Part model, mm, in its own coordinate system. A direction names the side the tool comes from. Coordinates: 2 decimals unless noted, no trailing zeros. Loops run counter-clockwise (first coordinate to the right, second up) from the corner with the lowest first, then second, coordinate; pieces in that order, holes last. Notation, with made-up numbers: M 28.5,43 L 32.5,43 A20 cw 32.5,68 Z; hole C 87.5,-18 d9. An arc over 180 degrees is marked long. Use a Markdown table: item, result. Add a question column.
1) Pin check, flat tips, straight feed: pin 1 Ø24 at (y, z) = (-2.5, -3.5) entering from +X; pin 2 Ø0.6 at (x, z) = (0.5, 8.5) entering from +Y; pin 3 Ø8 at (x, z) = (37.5, 14.5) entering from +Y; pin 4 Ø1.5 at (y, z) = (2.5, 9.5) entering from +X. Stop position of each tip, or through.
2) Tool access for faces 4 (the flat face through (65, 62, 0)), 5 (the flat face through (1, 0, -11.75)), 6 (the cylindrical face through (51.25, 63.48, 14.96)): list every direction of +Z, -Z, +X, -X, +Y, -Y with a clear straight run to the whole face (end or side of a thin tool).
3) Wall check: probe 1 along Y at (x, z) = (72, 18.5); probe 2 along X at (y, z) = (-5, -14); probe 3 along X at (y, z) = (30.5, 7). Give the ranges that are in metal, low to high. Write a range as from..to.
4) Pull direction X, two halves, no side cores. Call faces 1 (the flat face through (20, 5, -18)), 2 (the cylindrical face through (1.48, -11.75, -10.04)), 3 (the cylindrical face through (51.25, 63.48, -15.04)): released by +X, released by -X, zero draft, split by the parting line, or undercut.
5) Band-saw the part on B-B (z = -10). List the corners of the cut face in (x, y), plus the area to 3 significant figures.
6) Band-saw the part on C-C (x = 69.5). List the corners of the cut face in (y, z).
7) Band-saw the part on D-D (z = -2). List the corners of the cut face in (x, y), plus the area to 3 significant figures.
8) Band-saw the part on A-A (y = 9). List the corners of the cut face in (x, z), plus the area to 3 significant figures.
from build123d import *

# Parameters (mm, degrees)
SKETCH_1_W            = 30
SKETCH_1_H            = 30
EXTRUDE_1_DEPTH       = 3
EXTRUDE_2_DEPTH       = 30
EXTRUDE_3_DEPTH       = 40
FILLET_1_R            = 10
CUT_EXTRUDE_START     = -20
CUT_EXTRUDE_1_DEPTH   = 40
CUT_EXTRUDE_START_2   = -3
CUT_EXTRUDE_1_2_DEPTH = 3


# Read off the part's stored shape, not the designer's step: 切除-拉伸1
with BuildPart() as part:
    # 草图1 → 凸台-拉伸1 (new body)
    with BuildSketch(Plane(origin=(0, 0, 0), x_dir=(0, 0, -1), z_dir=(1, 0, 0))):
        Rectangle(SKETCH_1_W, SKETCH_1_H)
        with BuildLine():
            Line((-11.75, -10), (-11.75, 10))
            ThreePointArc((-11.75, 10), (-10, 11.75), (-8.25, 10))
            Line((-8.25, 10), (-8.25, -10))
            ThreePointArc((-8.25, -10), (-10, -11.75), (-11.75, -10))
        make_face(mode=Mode.SUBTRACT)
        with BuildLine():
            ThreePointArc((8.25, 10), (10, 11.75), (11.75, 10))
            Line((11.75, 10), (11.75, -10))
            ThreePointArc((11.75, -10), (10, -11.75), (8.25, -10))
            Line((8.25, -10), (8.25, 10))
        make_face(mode=Mode.SUBTRACT)
    extrude(amount=EXTRUDE_1_DEPTH)

    # 草图2 → 凸台-拉伸2 (add)
    with BuildSketch(Plane.XZ.offset(15)):
        Polygon((20, -20), (20, -15), (3, -15), (0, -15), (0, -20), align=None)
        Polygon((20, 20), (0, 20), (0, 15), (3, 15), (20, 15), align=None)
    extrude(amount=-EXTRUDE_2_DEPTH)

    # 草图3 → 凸台-拉伸3 (add)
    with BuildSketch(Plane.XY.offset(20)):
        with BuildLine():
            ThreePointArc((50, 65), (21.901058366, 48.400183617), (10.029526833, 18))
            Line((10.029526833, 18), (0, 18))
            Line((0, 18), (0, 15))
            Line((0, 15), (20, 15))
            ThreePointArc((20, 15), (26.843467388, 43.706297412), (50, 62))
            Line((50, 62), (80, 62))
            Line((80, 62), (80, 65))
            Line((80, 65), (50, 65))
        make_face()
    extrude(amount=-EXTRUDE_3_DEPTH)

    # 圆角1
    fillet_1_edges = [part.edges().sort_by_distance(p)[0] for p in [
        (10.029526833, 18, 0),
    ]]
    fillet(fillet_1_edges, radius=FILLET_1_R)

    # 切除-拉伸1 outline → 切除-拉伸1 (cut)
    with BuildSketch(Plane.XY.offset(CUT_EXTRUDE_START)):
        with BuildLine():
            Line((20, -15), (20, -5))
            ThreePointArc((20, -5), (17.071067812, -12.071067812), (10, -15))
            Line((10, -15), (20, -15))
        make_face()
    extrude(amount=CUT_EXTRUDE_1_DEPTH, mode=Mode.SUBTRACT)

    # Cut-Extrude 1 2 outline → Cut-Extrude 1 2 (cut)
    with BuildSketch(Plane(origin=(0, 65, 0), x_dir=(1, 0, 0), z_dir=(0, 1, 0)).offset(CUT_EXTRUDE_START_2)):
        with BuildLine():
            Line((75, 16.75), (53, 16.75))
            ThreePointArc((53, 16.75), (51.25, 15), (53, 13.25))
            Line((53, 13.25), (75, 13.25))
            ThreePointArc((75, 13.25), (76.75, 15), (75, 16.75))
        make_face()
        with BuildLine():
            Line((75, -13.25), (53, -13.25))
            ThreePointArc((53, -13.25), (51.25, -15), (53, -16.75))
            Line((53, -16.75), (75, -16.75))
            ThreePointArc((75, -16.75), (76.75, -15), (75, -13.25))
        make_face()
    extrude(amount=CUT_EXTRUDE_1_2_DEPTH, mode=Mode.SUBTRACT)


solid = part.part
Entries:
| question | item | result |
|---|---|---|
| 1 | pin 1 | x = 20 |
| 1 | pin 2 | y = 18 |
| 1 | pin 3 | y = 62.46 |
| 1 | pin 4 | through |
| 2 | face 4 | +Z, -Z, +X, -Y |
| 2 | face 5 | +X, -X |
| 2 | face 6 | +Y, -Y |
| 3 | probe 1 | 62..65 |
| 3 | probe 2 | 0..3 |
| 3 | probe 3 | 12.14..21.14 |
| 4 | face 1 | released by +X |
| 4 | face 2 | zero draft |
| 4 | face 3 | undercut |
| 5 | outline | M 0,-15 L 3,-15 L 3,-11.75 L 0,-11.75 Z; M 0,11.75 L 3,11.75 L 3,15 L 20,15 A45 cw 50,62 L 80,62 L 80,65 L 50,65 A50 ccw 11,26 A10 cw 1.2,18 L 0,18 Z |
| 5 | area | 589 mm2 |
| 6 | outline | M 62,-20 L 65,-20 L 65,-16.75 L 62,-16.75 Z; M 62,-13.25 L 65,-13.25 L 65,13.25 L 62,13.25 Z; M 62,16.75 L 65,16.75 L 65,20 L 62,20 Z |
| 7 | outline | M 0,-15 L 3,-15 L 3,15 L 20,15 A45 cw 50,62 L 80,62 L 80,65 L 50,65 A50 ccw 11,26 A10 cw 1.2,18 L 0,18 Z |
| 7 | area | 659 mm2 |
| 8 | outline | M 0,-20 L 20,-20 L 20,-15 L 3,-15 L 3,-11.75 L 0,-11.75 Z; M 0,-8.25 L 3,-8.25 L 3,8.25 L 0,8.25 Z; M 0,11.75 L 3,11.75 L 3,15 L 20,15 L 20,20 L 0,20 Z |
| 8 | area | 269 mm2 |
